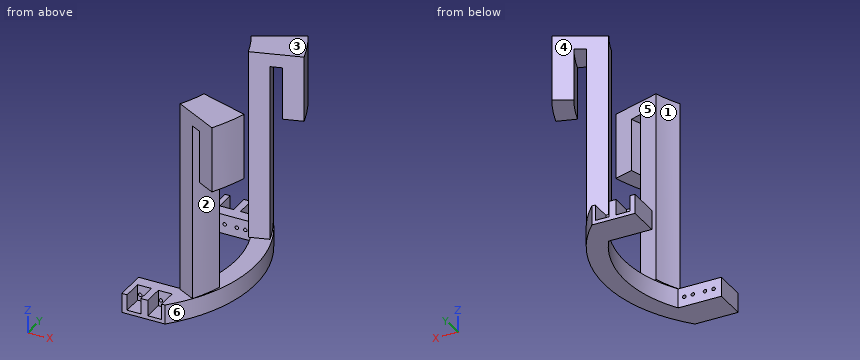
from build123d import *

# Parameters (mm, degrees)
F1_ANGLE_BACK = 28
F1_ANGLE      = 56
F2_ANGLE_BACK = 17
F2_ANGLE      = 34
F4_DEPTH      = 5.6388
F6_DEPTH      = 4.572
F7_R          = 0.508
F8_DEPTH      = 99.568
F9_R          = 0.508
F10_DEPTH     = 72.39


with BuildPart() as f1:
    # F0 (on Front) → F1 (revolve)
    with BuildSketch(Plane.XZ, mode=Mode.PRIVATE) as f1_sk:
        Polygon((0, 0), (0, 51.308), (3.2766, 51.308), (3.2766, 36.068), (8.9154, 36.068), (8.9154, 55.118), (-5.6388, 55.118), (-5.6388, 0), align=None)
    revolve(f1_sk.sketch.rotate(Axis((-46.7614, 0, 20.3579571098), (0, 0, 1)), -F1_ANGLE_BACK), axis=Axis((-46.7614, 0, 20.3579571098), (0, 0, 1)), revolution_arc=F1_ANGLE)

    # F0 (on Front) → F2 (revolve, cut)
    with BuildSketch(Plane.XZ, mode=Mode.PRIVATE) as f2_sk:
        Polygon((0, 0), (0, 51.308), (3.2766, 51.308), (3.2766, 36.068), (8.9154, 36.068), (8.9154, 55.118), (-5.6388, 55.118), (-5.6388, 0), align=None)
    revolve(f2_sk.sketch.rotate(Axis((-46.7614, 0, 20.3579571098), (0, 0, -1)), -F2_ANGLE_BACK), axis=Axis((-46.7614, 0, 20.3579571098), (0, 0, -1)), revolution_arc=F2_ANGLE, mode=Mode.SUBTRACT)

    # F3 (on Top) → F4 (join)
    with BuildSketch(Plane.XY):
        with BuildLine():
            Line((-22.6634080678, -28.1140467498), (-10.1666593224, -28.0782552096))
            ThreePointArc((-10.1666593224, -28.0782552096), (0.9017854761, 0.1178501934), (-10.3279875482, 28.2500919806))
            Line((-10.3279875482, 28.2500919806), (-22.8247362936, 28.2143004404))
            Line((-22.8247362936, 28.2143004404), (-22.7984871846, 19.0493268453))
            Line((-22.7984871846, 19.0493268453), (-10.3017384392, 19.0851183855))
            ThreePointArc((-10.3017384392, 19.0851183855), (-4.7369913968, 0.1017003521), (-10.1929084315, -18.9132816145))
            Line((-10.1929084315, -18.9132816145), (-22.6896571769, -18.9490731547))
            Line((-22.6896571769, -18.9490731547), (-22.6634080678, -28.1140467498))
        make_face()
    extrude(amount=-F4_DEPTH)

    # F5 (on face) → F6 (cut)
    with BuildSketch(Plane.XY):
        Polygon((-21.1558706034, -22.363909105), (-21.1394143184, -28.1096819278), (-17.151630674, -28.0982606436), (-17.168086959, -22.3524878208), align=None)
        Polygon((-15.161486959, -22.3524878208), (-15.1450471338, -28.0925136516), (-11.1572634894, -28.0810923674), (-11.1737033147, -22.3410665366), align=None)
        Polygon((-17.2965026148, 22.4843137237), (-17.3129588998, 28.2300865465), (-21.3007425442, 28.2186652623), (-21.2842862592, 22.4728924395), align=None)
        Polygon((-11.3021189705, 22.4957350078), (-11.3185917152, 28.2472548227), (-15.3063753596, 28.2358335385), (-15.2899026148, 22.4843137237), align=None)
    extrude(amount=-F6_DEPTH, mode=Mode.SUBTRACT)

    # F7 (on face) → F8 (cut)
    with BuildSketch(Plane(origin=(-0.0645214991, 22.527920253, 0), x_dir=(-0.9999958986, -0.0028640564, 0), z_dir=(-0.0028640564, 0.9999958986, 0))):
        with Locations((11.9996435616, -2.8194)):
            Circle(F7_R)
        with Locations((14.4888435616, -2.8194)):
            Circle(F7_R)
    extrude(amount=-F8_DEPTH, mode=Mode.SUBTRACT)

    # F9 (on face) → F10 (cut)
    with BuildSketch(Plane(origin=(-0.0645379589, 22.533667245, 0), x_dir=(-0.9999958986, -0.0028640564, 0), z_dir=(-0.0028640564, 0.9999958986, 0))):
        with Locations((17.9940353317, -2.8194)):
            Circle(F9_R)
        with Locations((20.4832353317, -2.8194)):
            Circle(F9_R)
    extrude(amount=-F10_DEPTH, mode=Mode.SUBTRACT)


solid = f1.part
Could you check a few things on this model? Use its own coordinates, in mm. Face numbers are marked on the shaded views. A direction names the side the tool comes from. Coordinates: 2 decimals unless noted, no trailing zeros. Order: outer loops, then holes, each group sorted by start corner. A loop starts at its lowest first (then second) coordinate and runs counter-clockwise, first axis right, second up. Notation, with made-up numbers: (65, 67) - (97, 67) arc R28 cw to (97, 86) - close; hole circle Ø4 at (10.25, 35.5). An arc over 180 degrees is marked (long way). Answer in a Markdown table with one row per item. Add a question column.
(1) If we mould it in two halves opening along Z, with no side actions, what happens to the marked faces 1, 2 and 3? For each: released by +Z, released by -Z, zero draft, split by the parting line, or undercut.
(2) If we section it at D-D, the plane x = 4: Please give me the cut outline in (y, z).
(3) If we section it at C-C, the plane y = -17.5: Please give me the cut outline in (x, z).
(4) Will these pins go through, and if not, where does the flat tip stop? pin 1 (2 mm diameter, centred on x = -18.5, y = -25.5, fed in from +Z); pin 2 (8 mm diameter, centred on x = -12.5, z = 8, fed in from -Y); pin 3 (3 mm diameter, centred on x = -6.5, z = 13, fed in from -Y).
(5) If we section it at B-B, the plane x = -8.25: Please give me the cut outline in (y, z), then the cut area to 3 significant figures.
(6) If we section it at A-A, the plane z = 18.5: Please give me the cut outline in (x, y), then the cut area to 3 significant figures.
(7) On a 3-axis mill with a long thin cutter (end or side, diameter ignored), from which of +Z, -Z, +X, -X, +Y, -Y can I reach the whole of each face in a straight line? I mean the marked faces 4, 5 and 6. Say none if no direction works.
(8) I need wall thicknesses on L1, parallel to Z at x = -13, y = -21; L2, parallel to Z at x = -0.75, y = -18; L3, parallel to X at y = 17, z = 46. Which ranges of each line are inside material? Lowest first, please.
Results are:
| question | item | result |
|---|---|---|
| 1 | face 1 | zero draft |
| 1 | face 2 | undercut |
| 1 | face 3 | released by +Z |
| 2 | outline | (-22.87, 36.07) - (-15.52, 36.07) - (-15.52, 55.12) - (-22.87, 55.12) - close; (15.52, 36.07) - (22.87, 36.07) - (22.87, 55.12) - (15.52, 55.12) - close |
| 3 | outline | (-9.55, 0) - (-9.35, 0) - (-9.35, -5.64) - (-3, -5.64) - (-3, 0) - (-3.4, 0) - (-3.4, 51.31) - (0.12, 51.31) - (0.12, 36.07) - (6.09, 36.07) - (6.09, 55.12) - (-9.55, 55.12) - close |
| 4 | pin 1 | stops at z = -4.57 |
| 4 | pin 2 | stops at y = -20.34 |
| 4 | pin 3 | stops at y = -21.95 |
| 5 | outline | (-25.87, -5.64) - (-15.4, -5.64) - (-15.4, 0) - (-14.42, 0) - (-14.42, 55.12) - (-20.48, 55.12) - (-20.48, 0) - (-25.87, 0) - close; (14.42, 0) - (15.4, 0) - (15.4, -5.64) - (25.87, -5.64) - (25.87, 0) - (20.48, 0) - (20.48, 55.12) - (14.42, 55.12) - close |
| 5 | area | 786 mm2 |
| 6 | outline | (-10.45, -19.31) - (-5.47, -21.95) arc R46.76 ccw to (-2.04, -13.67) - (-7.44, -12.02) arc R41.12 cw to start; (-10.45, 19.31) arc R41.12 cw to (-7.44, 12.02) - (-2.04, 13.67) arc R46.76 ccw to (-5.47, 21.95) - close |
| 6 | area | 95.1 mm2 |
| 7 | face 4 | +Z, -X, +Y |
| 7 | face 5 | +Z, +X |
| 7 | face 6 | -Z, +X |
| 8 | L1 | z = -5.64 to 0 |
| 8 | L2 | z = 51.31 to 55.12 |
| 8 | L3 | x = -9.32 to -3.2, 0.3 to 6.26 |
